Source: CAD feature listing. Evaluate the final solid. Frame: model axes, mm. Face numbers are marked on the shaded views. A direction names the side the tool comes from. Coordinates: 2 decimals unless noted, no trailing zeros. Order: outer loops, then holes, each group sorted by start corner. A loop starts at its lowest first (then second) coordinate and runs counter-clockwise, first axis right, second up. Notation, with made-up numbers: (42.25, 6.5) -> (47.25, 6.5) arc R18 cw to (47.25, 36.5) -> close; hole circle Ø1 at (29.25, 10). An arc over 180 degrees is marked (long way). Write item = value, one per line. Start each with the question number.
Item 1: Section query D-D (z = 0.4). Output: boundary loops of the cut face in (x, y), then the cut area to 3 significant figures.
Item 2: Mould query, pull axis Y, two halves, no side actions, for the marked faces 1, 2 and 3. Classes: released by +Y, released by -Y, zero draft, split by the parting line, or undercut.
Item 3: Set-up query: the marked faces 4 and 5. Return all of +Z, -Z, +X, -X, +Y, -Y with unobstructed straight access to the full face (end or side cutting, diameter ignored); none if empty.
Item 4: Section query C-C (x = 3.5). Output: boundary loops of the cut face in (y, z).
Item 5: Contact query for flat-ended pins moving along their axis: pin 1 (2.5 mm diameter, centred on x = 10, y = 6, fed in from -Z); pin 2 (2 mm diameter, centred on x = 10.5, y = 5.5, fed in from -Z). Output: stop coordinate, or through.
Item 6: Section query B-B (z = -0.5). Output: boundary loops of the cut face in (x, y), then the cut area to 3 significant figures.
Item 7: Section query A-A (y = 5.5). Output: boundary loops of the cut face in (x, z).
Item 8: Ray query, line 1 along X through (y, z) = (7, -1.8); line 2 along Y through (x, z) = (10, 0.55); line 3 along X through (y, z) = (6.5, 0.45). Return the intervals inside material, ascending. Write a range as [from, to].
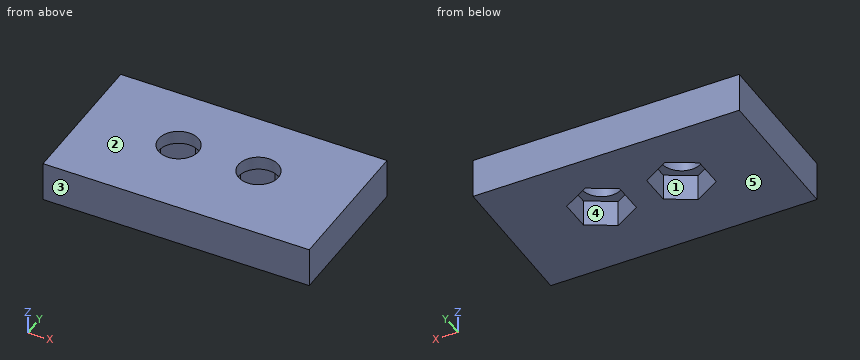
Autodesk Fusion 360 part; units mm, degrees
sketch "Sketch1" plane through (0, 0, 0) normal (0, 0, 1) x (1, 0, 0)
  line L0 (0, 0) -> (14, 0)
  line L1 (14, 0) -> (14, 11)
  line L2 (14, 11) -> (0, 11)
  line L3 (0, 11) -> (0, 0)
  dimension "d1" = 14
  dimension "d2" = 11
extrude "Extrude1" add sketch "Sketch1" along normal blind 2
sketch "Sketch2" plane through (0, 0, 0) normal (0, -1, 0) x (1, 0, 0)
  line L0 (0, 0) -> (14, 0)
  line L1 (14, 0) -> (14, 2)
  line L2 (14, 2) -> (0, 2)
  line L3 (0, 2) -> (0, 0)
sketch "Sketch3" plane through (0, 0, 2) normal (0, 0, 1) x (-1, 0, 0)
  line L0 (0, -11) -> (0, 0)
  line L1 (0, 0) -> (-14, 0)
  line L2 (-14, 0) -> (-14, -11)
  line L3 (-14, -11) -> (0, -11)
  line L4 (0, -11) -> (3, -11)
  line L5 (3, -11) -> (3, 0)
  line L6 (3, 0) -> (0, 0)
  line L7 (0, 0) -> (0, -11)
  line L8 (-14, -11) -> (-17, -11)
  line L9 (-17, -11) -> (-17, 0)
  line L10 (-17, 0) -> (-14, 0)
  line L11 (-14, 0) -> (-14, -11)
  dimension "d26" = 3
  dimension "d27" = 3
extrude "Extrude2" add sketch "Sketch3" along normal blind 7 and the other way blind 2 contours L0 L4 L5 L6 L7 | L2 L8 L9 L10 L11
sketch "Sketch4" plane through (0, 0, 0) normal (0, 0, -1) x (1, 0, 0)
  line L0 (-3, -11) -> (17, -11)
  line L1 (17, -11) -> (17, 0)
  line L2 (17, 0) -> (-3, 0)
  line L3 (-3, 0) -> (-3, -11)
  line L4 (-3, 0) -> (17, 0)
  line L5 (17, 0) -> (17, -11)
  line L6 (17, -11) -> (-3, -11)
  line L7 (-3, -11) -> (-3, 0)
extrude "Extrude3" add sketch "Sketch4" along normal blind 2
sketch "Sketch5" plane through (0, 0, 2) normal (0, 0, 1) x (-1, 0, 0)
  line L0 (0, -11) -> (0, 0)
  line L1 (0, 0) -> (-14, 0)
  line L2 (-14, 0) -> (-14, -11)
  line L3 (-14, -11) -> (0, -11)
  line L4 (-7, -11) -> (-7, -6)
  line L5 (-7, -6) -> (0, -6)
  line L6 (-7, -6) -> (-14, -6)
  circle A0 centre (-4, -6) radius 1.5
  circle A1 centre (-10, -6) radius 1.5
  dimension "d11" = 5
  dimension "d12" = 3
  dimension "d13" = 3
  dimension "d31" = 6
  dimension "d32" = 4
extrude "Extrude4" cut sketch "Sketch5" against normal blind 4 contours L5 A0 | L5 A0 | L6 A1 | L6 A1
sketch "Sketch7" plane through (0, 0, -2) normal (0, 0, -1) x (1, 0, 0)
  circle A0 centre (4, -6) radius 1.5
  circle A1 centre (10, -6) radius 1.5
  line L0 (-3, -11) -> (17, -11)
  line L1 (17, -11) -> (17, 0)
  line L2 (17, 0) -> (-3, 0)
  line L3 (-3, 0) -> (-3, -11)
  line L4 (11.9876, -4.8242) -> (9.9755, -3.6907)
  line L5 (9.9755, -3.6907) -> (7.9879, -4.8666)
  line L6 (7.9879, -4.8666) -> (8.0124, -7.1758)
  line L7 (8.0124, -7.1758) -> (10.0245, -8.3093)
  line L8 (10.0245, -8.3093) -> (12.0121, -7.1334)
  line L9 (12.0121, -7.1334) -> (11.9876, -4.8242)
  line L10 (2.0156, -7.1814) -> (4.0309, -8.3092)
  line L11 (4.0309, -8.3092) -> (6.0153, -7.1278)
  line L12 (6.0153, -7.1278) -> (5.9844, -4.8186)
  line L13 (5.9844, -4.8186) -> (3.9691, -3.6908)
  line L14 (3.9691, -3.6908) -> (1.9847, -4.8722)
  line L15 (1.9847, -4.8722) -> (2.0156, -7.1814)
  point P0 (10, -6)
  point P1 (4, -6)
  dimension "d22" = 2
  dimension "d23" = 2
extrude "Extrude6" cut sketch "Sketch7" against normal blind 2 contours L4 L5 L6 L7 L8 L9 | L10 L11 L12 L13 L14 L15
fillet "Fillet1" radius 1 4 edges at (-3, 5.5, 9) (0, 5.5, 9) (14, 5.5, 9) (17, 5.5, 9)
sketch "Sketch8" plane through (0, 11, 0) normal (0, 1, 0) x (-1, 0, 0)
  arc A0 (-16, 9) -> (-17, 8) centre (-16, 8) ccw
  line L0 (-17, 8) -> (-17, -2)
  line L1 (-17, -2) -> (3, -2)
  line L2 (3, -2) -> (3, 8)
  arc A1 (3, 8) -> (2, 9) centre (2, 8) ccw
  line L3 (2, 9) -> (1, 9)
  arc A2 (1, 9) -> (0, 8) centre (1, 8) ccw
  line L4 (0, 8) -> (0, 2)
  line L5 (0, 2) -> (-14, 2)
  line L6 (-14, 2) -> (-14, 8)
  arc A3 (-14, 8) -> (-15, 9) centre (-15, 8) ccw
  line L7 (-15, 9) -> (-16, 9)
  line L8 (-14, 2) -> (-17, 2)
  line L9 (-17, 2) -> (-17, 9)
  line L10 (-17, 9) -> (-14, 9)
  line L11 (-14, 9) -> (-14, 2)
  line L12 (0, 2) -> (3, 2)
  line L13 (3, 2) -> (3, 9)
  line L14 (3, 9) -> (0, 9)
  line L15 (0, 9) -> (0, 2)
extrude "Extrude7" cut sketch "Sketch8" against normal blind 4 contours A0 L0 L6 A3 L7 L8 L9 L10 L11 | L2 A1 L3 A2 L4 L12 L13 L14 L15
fillet "Fillet2" radius 2 1 edges at (7, 11, 2)
delete_face "DeleteFace1" 1 faces at (10.3333, 9.0952, 1.9977)
sketch "Sketch9" plane through (17, 0, 0) normal (1, 0, 0) x (0, 1, 0)
  line L0 (11, 2) -> (7, 2)
  line L1 (7, 2) -> (7, 8)
  line L2 (7, 8) -> (0, 8)
  line L3 (0, 8) -> (0, -2)
  line L4 (0, -2) -> (11, -2)
  line L5 (11, -2) -> (11, 2)
  line L6 (7, 2) -> (0, 2)
  line L7 (0, 2) -> (0, 9)
  line L8 (0, 9) -> (7, 9)
  line L9 (7, 9) -> (7, 2)
extrude "Extrude8" cut sketch "Sketch9" against normal blind 20 contours L1 L2 L3 L6 L7 L9 | L2 L7 L8 L9
extrude "Extrude9" cut 1 faces at (7.8887, 1.5125, 2) along direction (0, 0, -1) blind 1
Computed:
q1.outline = (-3, 0) -> (17, 0) -> (17, 11) -> (-3, 11) -> close; hole circle Ø3 at (4, 6); hole circle Ø3 at (10, 6)
q1.area = 206 mm^2
q2.face_1 = undercut
q2.face_2 = zero draft
q2.face_3 = released by -Y
q3.face_4 = -Z
q3.face_5 = -Z, +X, -X, +Y, -Y
q4.outline = (0, -2) -> (3.97, -2) -> (3.97, 0) -> (4.59, 0) -> (4.59, 1) -> (0, 1) -> close; (7.41, 0) -> (8.01, 0) -> (8.01, -2) -> (11, -2) -> (11, 1) -> (7.41, 1) -> close
q5.pin_1 = through
q5.pin_2 = 0
q6.outline = (-3, 0) -> (17, 0) -> (17, 11) -> (-3, 11) -> close; hole (1.98, 4.87) -> (3.97, 3.69) -> (5.98, 4.82) -> (6.02, 7.13) -> (4.03, 8.31) -> (2.02, 7.18) -> close; hole (7.99, 4.87) -> (9.98, 3.69) -> (11.99, 4.82) -> (12.01, 7.13) -> (10.02, 8.31) -> (8.01, 7.18) -> close
q6.area = 192 mm^2
q7.outline = (-3, -2) -> (1.99, -2) -> (1.99, 0) -> (2.59, 0) -> (2.59, 1) -> (-3, 1) -> close; (5.41, 0) -> (5.99, 0) -> (5.99, -2) -> (7.99, -2) -> (7.99, 0) -> (8.59, 0) -> (8.59, 1) -> (5.41, 1) -> close; (11.41, 0) -> (11.99, 0) -> (11.99, -2) -> (17, -2) -> (17, 1) -> (11.41, 1) -> close
q8.line_1 = [-3, 2.01], [6.01, 8.01], [12.01, 17]
q8.line_2 = [0, 4.5], [7.5, 11]
q8.line_3 = [-3, 2.59], [5.41, 8.59], [11.41, 17]
